```python
from build123d import *

# Parameters (mm, degrees)
F0_R     = 1.6002
F1_DEPTH = 9.525
F0_R_2   = 11.1125
F2_DEPTH = 3.175
F3_R     = 0.254
F4_R     = 2.286
F4_R_2   = 1.6002
F5_DEPTH = 6.35
F6_R     = 2.286
F6_R_2   = 1.6002
F7_DEPTH = 5.842


with BuildPart() as f1:
    # F0 (on Top) → F1 (new body)
    with BuildSketch(Plane.XY):
        Circle(F0_R)
    extrude(amount=F1_DEPTH)

    # F0 (on Top) → F2 (join)
    with BuildSketch(Plane.XY):
        Circle(F0_R_2)
        Circle(F0_R, mode=Mode.SUBTRACT)
    extrude(amount=F2_DEPTH)

    # F3
    f3_edges = [f1.edges().sort_by_distance(p)[0] for p in [
        (-11.1125, 0, 0),
    ]]
    fillet(f3_edges, radius=F3_R)

    # F4 (on face) → F5 (join)
    with BuildSketch(Plane.XY.offset(9.525)):
        Circle(F4_R)
        Circle(F4_R_2, mode=Mode.SUBTRACT)
    extrude(amount=-F5_DEPTH)

    # F6 (on face) → F7 (cut)
    with BuildSketch(Plane.XY.offset(9.525)):
        Circle(F6_R)
        Circle(F6_R_2, mode=Mode.SUBTRACT)
    extrude(amount=-F7_DEPTH, mode=Mode.SUBTRACT)


solid = f1.part
```
Build history of the part. All positions in model axes, mm. A direction names the side the tool comes from. Give positions to 0.01 mm unless a question says otherwise; leave off trailing zeros. Loops run counter-clockwise (first coordinate to the right, second up) from the corner with the lowest first, then second, coordinate; pieces in that order, holes last. Notation, with made-up numbers: (-19, 41) -> (11, 41) arc R9 cw to (11, 46) -> close; hole circle Ø4 at (60.25, -37.5). An arc over 180 degrees is marked (long way). One line per question, with ' | ' between items. Start each with the question number.
1) Cut at C-C (z = 1). Give the cut face in (x, y) (1 decimal), plus the area to 3 significant figures.
2) Pin check, flat tips, straight feed: pin 1 (2 mm diameter, centred on x = -4.5, z = 8.5, fed in from +Y); pin 2 (3 mm diameter, centred on x = -0.5, y = -5.5, fed in from +Z) (3 decimals). Stop position of each tip, or through.
3) Cut at D-D (z = 6.25). Give the cut face in (x, y).
4) 3-axis set-ups, long thin cutter, end or side, ignore diameter. For faces 1 (the flat face through (0, 0, 0)), 2 (the flat face through (0, 2, 3.683)): which of +Z, -Z, +X, -X, +Y, -Y reach the whole face in a straight line?
5) Probe L1, parallel to Z at x = -2.5, y = -3.25 (3 decimals); L2, parallel to Y at x = 8.5, z = 2.25; L3, parallel to X at y = 6.25, z = 0.5. List the from-to ranges inside material, lowest first.
Return value:
1) outline: circle Ø22.2 at (0, 0) | area: 388 mm^2
2) pin 1: through | pin 2: z = 3.175
3) outline: circle Ø3.2 at (0, 0)
4) face 1: -Z, +X, -X, +Y, -Y | face 2: +Z
5) L1: 0 to 3.175 | L2: -7.16 to 7.16 | L3: -9.19 to 9.19
